from build123d import *

# Parameters (mm, degrees)
PAD_DEPTH   = 3
FILLET_R    = 1
FILLET001_R = 1
FILLET002_R = 1
FILLET003_R = 1
FILLET004_R = 1
FILLET005_R = 1


with BuildPart() as part:
    # Sketch → Pad (new body)
    with BuildSketch(Plane.XY):
        Polygon((-10, 15.751367), (10, 15.751367), (10, -14.248633), (-40, -14.248633), (-40, -4.248633), (-25, -4.248633), (-25, 5.751367), (-10, 5.751367), align=None)
    extrude(amount=PAD_DEPTH)

    # Fillet
    fillet_edges = [part.edges().sort_by_distance(p)[0] for p in [
        (-40, -4.248633, 1.5),
    ]]
    fillet(fillet_edges, radius=FILLET_R)

    # Fillet001
    fillet001_edges = [part.edges().sort_by_distance(p)[0] for p in [
        (-25, -4.248633, 1.5),
    ]]
    fillet(fillet001_edges, radius=FILLET001_R)

    # Fillet002
    fillet002_edges = [part.edges().sort_by_distance(p)[0] for p in [
        (-25, 5.751367, 1.5),
    ]]
    fillet(fillet002_edges, radius=FILLET002_R)

    # Fillet003
    fillet003_edges = [part.edges().sort_by_distance(p)[0] for p in [
        (-10, 5.751367, 1.5),
    ]]
    fillet(fillet003_edges, radius=FILLET003_R)

    # Fillet004
    fillet004_edges = [part.edges().sort_by_distance(p)[0] for p in [
        (-10, 15.751367, 1.5),
    ]]
    fillet(fillet004_edges, radius=FILLET004_R)

    # Fillet005
    fillet005_edges = [part.edges().sort_by_distance(p)[0] for p in [
        (10, 15.751367, 1.5),
    ]]
    fillet(fillet005_edges, radius=FILLET005_R)


solid = part.part
Read the model definition and answer for the solid it produces. Units are mm, in the model's axes. A direction names the side the tool comes from. Round coordinates to 2 decimals unless told otherwise and drop trailing zeros. Loops run counter-clockwise (first coordinate to the right, second up) from the corner with the lowest first, then second, coordinate; pieces in that order, holes last. Notation, with made-up numbers: (18.25, -19) - (76.25, -19) arc R10 cw to (76.25, -4) - close; hole circle Ø6 at (75, -36.5). An arc over 180 degrees is marked (long way). One line per question, with ' | ' between items. Start each with the question number.
Q1. For faces 1 (the flat face through (-33, -4.249, 1)), 2 (the flat face through (-9, -2, 3)), determine the directions among +Z, -Z, +X, -X, +Y, -Y from which every point of the face is accessible in a straight line to the end or side of a thin tool.
Q2. Section B-B on x = -26.5 is taken. Give the vertices of the cut face in (y, z), plus the area to 3 significant figures.
Q3. Section C-C on y = 13 is taken. Give the vertices of the cut face in (x, z), plus the area to 3 significant figures.
Q4. Find the intervals of material crossed by L1, parallel to Y at x = -13, z = 1.1; L2, parallel to X at y = 3.25, z = 1.25; L3, parallel to X at y = 7.75, z = 2.5, in increasing order.
Q5. Section A-A on z = 0.55 is taken. Give the vertices of the cut face in (x, y).
Q6. Flat-ended cylindrical pins translate along their axes: pin 1 (0.9 mm diameter, centred on y = -0.5, z = 2, fed in from -X); pin 2 (1.5 mm diameter, centred on x = -10, y = 7.5, fed in from -Z); pin 3 (1.5 mm diameter, centred on x = -20, z = 2, fed in from +Y); pin 4 (0.9 mm diameter, centred on x = -30, z = 1, fed in from +Y). Find the tip coordinate at first contact, or state that the pin passes through.
Established:
1) face 1: +Z, -Z, -X, +Y | face 2: +Z, +X, -X, +Y, -Y
2) outline: (-14.25, 0) - (-4.25, 0) - (-4.25, 3) - (-14.25, 3) - close | area: 30.0 mm²
3) outline: (-10, 0) - (10, 0) - (10, 3) - (-10, 3) - close | area: 60.0 mm²
4) L1: -14.25 to 5.75 | L2: -25 to 10 | L3: -10 to 10
5) outline: (-40, -14.25) - (10, -14.25) - (10, 14.75) arc R1 ccw to (9, 15.75) - (-9, 15.75) arc R1 ccw to (-10, 14.75) - (-10, 6.75) arc R1 cw to (-11, 5.75) - (-24, 5.75) arc R1 ccw to (-25, 4.75) - (-25, -3.25) arc R1 cw to (-26, -4.25) - (-39, -4.25) arc R1 ccw to (-40, -5.25) - close
6) pin 1: x = -25 | pin 2: z = 0 | pin 3: y = 5.75 | pin 4: y = -4.25
